Here's how the part is built. I have some questions about the finished solid (model axes, mm). Face numbers are marked on the shaded views. Coordinates: 2 decimals unless noted, no trailing zeros. Write each loop counter-clockwise with the first axis right and the second up, starting at its lowest first coordinate (ties: lowest second). Pieces come first, ordered by that corner, then holes. Notation, with made-up numbers: M -17,40.25 L 32,40.25 A27 cw 32,68.25 Z; hole C 70.25,40.5 d2. An arc over 180 degrees is marked long. Use one line per item in the form item = value. Start each with the question number.
1. I'm going to push flat-ended pins straight in: pin 1 Ø2 at (x, z) = (38, 5) entering from -Y; pin 2 Ø3 at (y, z) = (-12, 2) entering from -X; pin 3 Ø5 at (x, z) = (39.49, 3.5) entering from +Y. Where does each tip first touch, or does it pass through?
2. I want a section at A-A, the plane x = -39. List the corners of the cut face in (y, z) for me, plus the area to 3 significant figures.
3. I want a section at B-B, the plane y = -16. List the corners of the cut face in (x, z) for me.
4. I want a section at D-D, the plane x = 0. List the corners of the cut face in (y, z) for me, plus the area to 3 significant figures.
5. Please list where these lines run through material, in increasing order: line 1 along Y through (x, z) = (-1, 4); line 2 along X through (y, z) = (-10, 6); line 3 along Z through (x, y) = (33, -6.5). Write a range as [from, to].
6. Thinking about a two-plate mould opening in X: for the marked faces 1, 2, 3 and 4, which applies, released by +X, released by -X, zero draft, split by the parting line, or undercut?
from build123d import *

# Parameters (mm, degrees)
BOSS_EXTRUDE2_DEPTH      = 7
BOSS_EXTRUDE7_DEPTH      = 3.5
BOSS_EXTRUDE7_DEPTH_BACK = 3.2
SKETCH7_W                = 10
SKETCH7_H                = 10
SKETCH8_R                = 1.5
CUT_EXTRUDE3_DEPTH       = 10
FILLET1_R                = 5
FILLET2_R                = 5
FILLET3_R                = 5
SKETCH9_W                = 8
SKETCH9_H                = 3
BOSS_EXTRUDE8_DEPTH      = 7
SKETCH10_R               = 1.5
CUT_EXTRUDE4_DEPTH       = 10
FILLET4_R                = 2
FILLET5_R                = 2
CUT_EXTRUDE5_DEPTH       = 7


with BuildPart() as part:
    # Sketch1 → Boss-Extrude2 (new body)
    with BuildSketch(Plane.XY):
        with BuildLine():
            Line((36, 0), (31, 0))
            ThreePointArc((31, 0), (30.997217748, -0.415321451), (30.98887149, -0.830568352))
            ThreePointArc((30.98887149, -0.830568352), (29.746163614, -2.974229152), (30.539836631, -5.321501534))
            ThreePointArc((30.539836631, -5.321501534), (0.032857513, -30.999982587), (-30.528487289, -5.386229095))
            ThreePointArc((-30.528487289, -5.386229095), (-29.731741507, -3.029439038), (-30.987456583, -0.881779181))
            ThreePointArc((-30.987456583, -0.881779181), (-30.996863987, -0.440934196), (-31, 0))
            Line((-31, 0), (-36, 0))
            ThreePointArc((-36, 0), (0, -36), (36, 0))
        make_face()
    extrude(amount=BOSS_EXTRUDE2_DEPTH)

    # Sketch7 → Boss-Extrude7 (add, two sides: drawn at the far end of the back side and taken through both)
    with BuildSketch(Plane(origin=(0, 0, 0), x_dir=(-1, 0, 0), z_dir=(0, 0, -1)).offset(-BOSS_EXTRUDE7_DEPTH_BACK)):
        with Locations((38, 0.5)):
            Rectangle(SKETCH7_W, SKETCH7_H)
    extrude(amount=BOSS_EXTRUDE7_DEPTH + BOSS_EXTRUDE7_DEPTH_BACK)

    # Sketch8 → Cut-Extrude3 (cut)
    with BuildSketch(Plane.XY.offset(3.2)):
        with Locations((-39, -0.8)):
            Circle(SKETCH8_R)
    extrude(amount=-CUT_EXTRUDE3_DEPTH, mode=Mode.SUBTRACT)

    # Fillet1
    fillet1_edges = [part.edges().sort_by_distance(p)[0] for p in [
        (-43, 5.5, -0.15),
    ]]
    fillet(fillet1_edges, radius=FILLET1_R)

    # Fillet2
    fillet2_edges = [part.edges().sort_by_distance(p)[0] for p in [
        (-43, -4.5, -0.15),
    ]]
    fillet(fillet2_edges, radius=FILLET2_R - 0.0001)  # a hair under: the kernel refuses the full size

    # Fillet3
    fillet3_edges = [part.edges().sort_by_distance(p)[0] for p in [
        (-33, 5.5, -0.15),
    ]]
    fillet(fillet3_edges, radius=FILLET3_R - 0.0001)  # a hair under: the kernel refuses the full size

    # Sketch9 → Boss-Extrude8 (add)
    with BuildSketch(Plane.XY.offset(7)):
        with Locations((39, -2.5)):
            Rectangle(SKETCH9_W, SKETCH9_H)
    extrude(amount=-BOSS_EXTRUDE8_DEPTH)

    # Sketch10 → Cut-Extrude4 (cut)
    with BuildSketch(Plane(origin=(0, -1, 0), x_dir=(1, 0, 0), z_dir=(0, 1, 0))):
        with Locations(Location((39.486108431, -3.5, 0), (0, 0, 180))):
            Circle(SKETCH10_R)
    extrude(amount=-CUT_EXTRUDE4_DEPTH, mode=Mode.SUBTRACT)

    # Fillet4
    fillet4_edges = [part.edges().sort_by_distance(p)[0] for p in [
        (43, -2.5, 7),
    ]]
    fillet(fillet4_edges, radius=FILLET4_R)

    # Fillet5
    fillet5_edges = [part.edges().sort_by_distance(p)[0] for p in [
        (43, -2.5, 0),
    ]]
    fillet(fillet5_edges, radius=FILLET5_R)

    # Sketch11 → Cut-Extrude5 (cut)
    with BuildSketch(Plane(origin=(0, 0, -3.5), x_dir=(-1, 0, 0), z_dir=(0, 0, -1))):
        with BuildLine():
            Line((33, 0.5), (33, 0.179462338))
            Line((33, 0.179462338), (40.279801287, 4.950000684))
            ThreePointArc((40.279801287, 4.950000684), (39.17260321, 5.3605557), (38, 5.5))
            ThreePointArc((38, 5.5), (34.464466094, 4.035533906), (33, 0.5))
        make_face()
    extrude(amount=-CUT_EXTRUDE5_DEPTH, mode=Mode.SUBTRACT)


with BuildPart() as cut_extrude5_kept_piece:
    # of the separate pieces the step leaves, the one the design keeps (cut_extrude5_pieces_kept)
    add(part.part.solids().sort_by_distance((43, -4, 2))[0])


solid = cut_extrude5_kept_piece.part
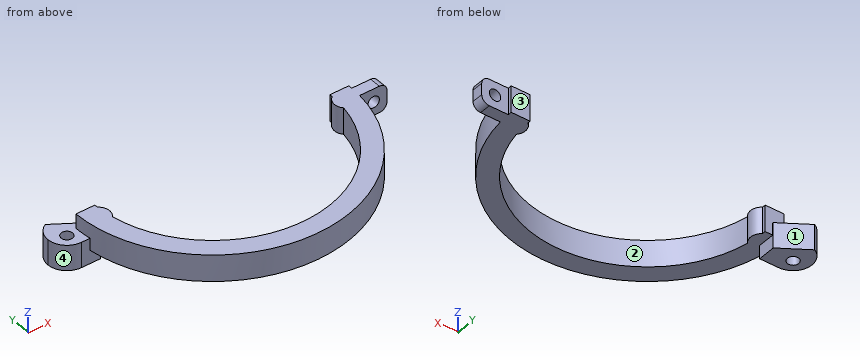
Answer list:
q1.pin_1 = -4
q1.pin_2 = -34.43
q1.pin_3 = -1
q2.outline = M -4.4,-3.5 L -2.3,-3.5 L -2.3,3.2 L -4.4,3.2 Z; M 0.7,-3.5 L 4.11,-3.5 L 4.11,3.2 L 0.7,3.2 Z
q2.area = 36.9 mm²
q3.outline = M -32.25,0 L -26.55,0 L -26.55,7 L -32.25,7 Z; M 26.55,0 L 32.25,0 L 32.25,7 L 26.55,7 Z
q4.outline = M -36,0 L -31,0 L -31,7 L -36,7 Z
q4.area = 35.0 mm²
q5.line_1 = [-35.99, -30.98]
q5.line_2 = [-34.58, -29.34], [29.34, 34.58]
q5.line_3 = [0, 7]
q6.face_1 = released by +X
q6.face_2 = undercut
q6.face_3 = zero draft
q6.face_4 = released by -X
